Check sheet for the drawn part. Datum: minimum x, y, z corner. Units: mm. Give positions to 0.01 mm unless a question says otherwise; leave off trailing zeros. Loops run counter-clockwise (first coordinate to the right, second up) from the corner with the lowest first, then second, coordinate; pieces in that order, holes last. Notation, with made-up numbers: (56.25, 53) - (89.25, 53) arc R27 ccw to (89.25, 74) - close; hole circle Ø6 at (50.25, -30.5). An arc over 180 degrees is marked (long way). Use a Markdown table: item, result. Add a question column.
1. Cross-section at C-C on x = 5. Enter the section's corners in (y, z), and give its area (3 significant figures).
2. Cross-section at D-D on y = 9. Enter the section's corners in (x, z).
3. Material ranges on L1, parallel to Z at x = 5, y = 3.55; L2, parallel to Y at x = 3.75, z = 6.75; L3, parallel to Z at x = 7, y = 4 (1 decimal), recorded low to high.
4. Depth check by flat-ended pin: P1, Ø5.5, axis at x = 5, z = 5, coming from the -Y side; P2, Ø1, axis at x = 7, y = 4.5, coming from the -Z side; P3, Ø4, axis at y = 1.5, z = 7.5, coming from the -X side (3 decimals). Enter the tip coordinate at first touch or a pass-through.
5. Cross-section at A-A on y = 2.5. Enter the section's corners in (x, z).
6. Cross-section at B-B on z = 5. Enter the section's corners in (x, y), and give its area (3 significant figures).
7. Draft check along Z on the marked faces 1, 2 and 3. Enter one of: pulls with the +Z half, pulls with the -Z half, needs draft (parallel to the pull), parting line crosses it, or undercut.
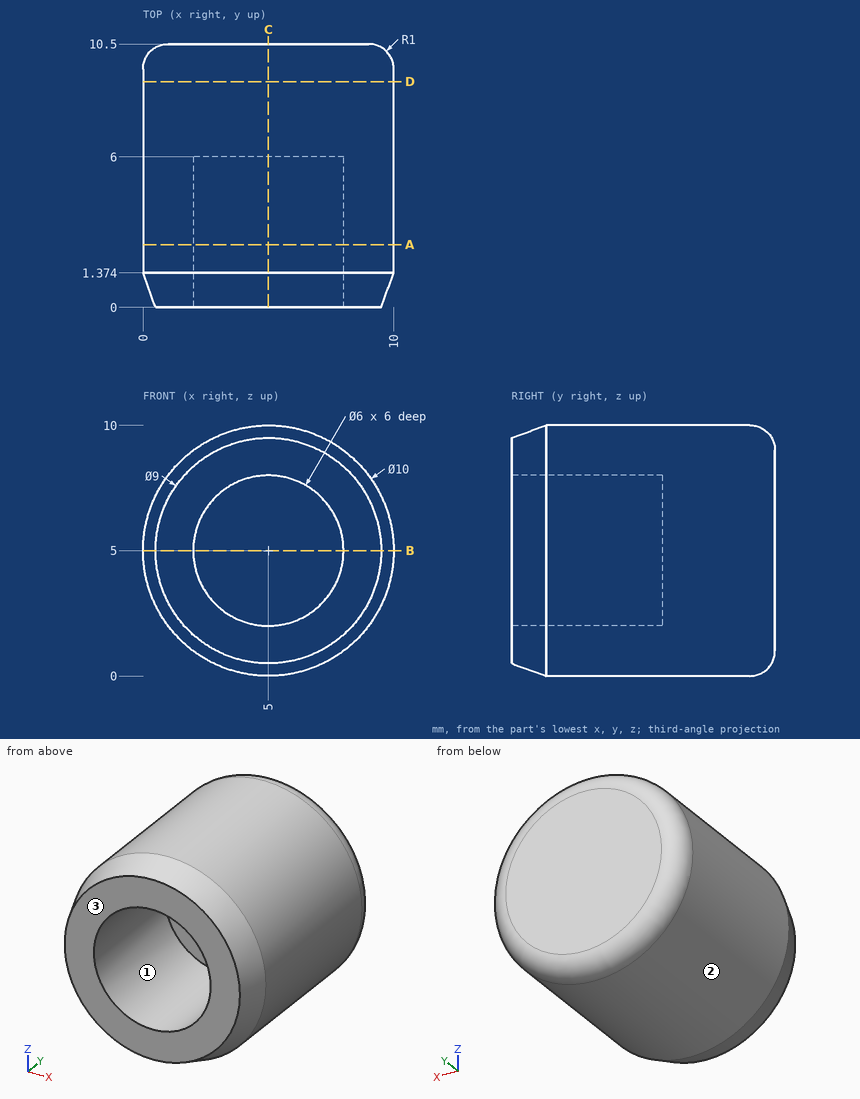
Values found:
| question | item | result |
|---|---|---|
| 1 | outline | (0, 0.5) - (1.37, 0) - (9.5, 0) arc R1 ccw to (10.5, 1) - (10.5, 9) arc R1 ccw to (9.5, 10) - (1.37, 10) - (0, 9.5) - (0, 8) - (6, 8) - (6, 2) - (0, 2) - close |
| 1 | area | 67.9 mm2 |
| 2 | outline | circle Ø10 at (5, 5) |
| 3 | L1 | z = 0 to 2, 8 to 10 |
| 3 | L2 | y = 6 to 10.5 |
| 3 | L3 | z = 0.4 to 2.8, 7.2 to 9.6 |
| 4 | P1 | stops at y = 6 |
| 4 | P2 | stops at z = 0.23 |
| 4 | P3 | stops at x = 0.025 |
| 5 | outline | circle Ø10 at (5, 5); hole circle Ø6 at (5, 5) |
| 6 | outline | (0, 1.37) - (0.5, 0) - (2, 0) - (2, 6) - (8, 6) - (8, 0) - (9.5, 0) - (10, 1.37) - (10, 9.5) arc R1 ccw to (9, 10.5) - (1, 10.5) arc R1 ccw to (0, 9.5) - close |
| 6 | area | 67.9 mm2 |
| 7 | face 1 | undercut |
| 7 | face 2 | parting line crosses it |
| 7 | face 3 | needs draft |
